Check sheet for the drawn part. Datum: minimum x, y, z corner. Units: mm. A direction names the side the tool comes from. Give positions to 0.01 mm unless a question says otherwise; leave off trailing zeros. Write each loop counter-clockwise with the first axis right and the second up, starting at its lowest first coordinate (ties: lowest second). Pieces come first, ordered by that corner, then holes.
(1) Cross-section at C-C (z = 51). Record the boundary of the cut face in (x, y).
(2) Cross-section at A-A (z = 5). Record the boundary of the cut face in (x, y), and give its area (3 significant figures).
(3) Thickness scan on line 1 along X through (y, z) = (1.55, 75); line 2 along Z through (x, y) = (5.25, 17.5); line 3 along Y through (x, z) = (6.25, 7.5). Record the ranges inside material, lowest first.
(4) Depth check by flat-ended pin: P1, Ø4.5, axis at y = 1, z = 13, coming from the -X side; P2, Ø1, axis at x = 8.5, y = 30, coming from the +Z side; P3, Ø8, axis at y = 33.5, z = 70, coming from the -X side. Enter the tip coordinate at first touch or a pass-through.
(5) Cross-section at D-D (y = 17). Record the boundary of the cut face in (x, z), and give its area (3 significant figures).
(6) Cross-section at B-B (x = 7.1). Record the boundary of the cut face in (y, z).
(7) Tool access check on the marked faces 1, 2 and 3. Record the directions out of +Z, -Z, +X, -X, +Y, -Y that give a thin tool (end or side, any length) a straight path to the whole face; none if there is none.
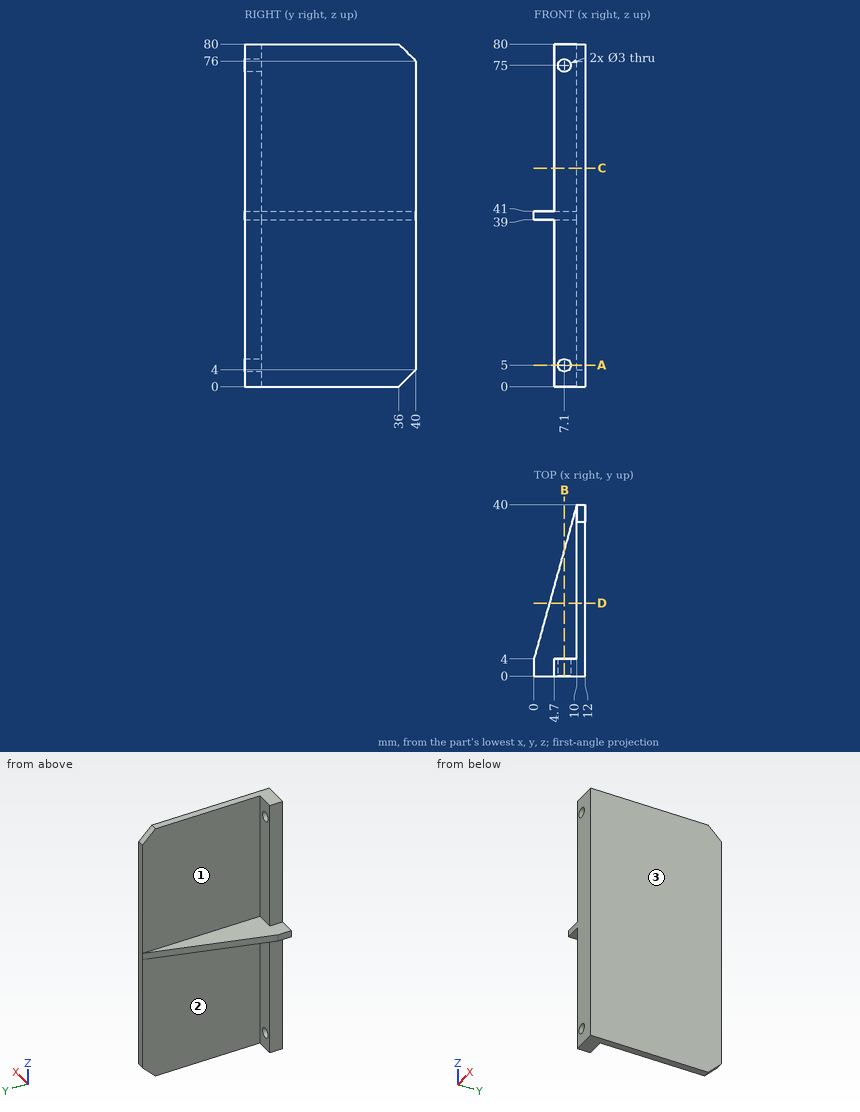
Reply:
1. outline: (4.7, 0) - (12, 0) - (12, 40) - (10, 40) - (10, 4) - (4.7, 4) - close
2. outline: (4.7, 0) - (5.6, 0) - (5.6, 4) - (4.7, 4) - close; (8.6, 0) - (12, 0) - (12, 40) - (10, 40) - (10, 4) - (8.6, 4) - close
2. area: 89.2 mm2
3. line 1: x = 4.7 to 5.6, 8.6 to 12
3. line 2: z = 39 to 41
3. line 3: y = 0 to 4
4. P1: stops at x = 4.7
4. P2: stops at z = 41
4. P3: stops at x = 10
5. outline: (3.61, 39) - (10, 39) - (10, 0) - (12, 0) - (12, 80) - (10, 80) - (10, 41) - (3.61, 41) - close
5. area: 173 mm2
6. outline: (0, 0) - (4, 0) - (4, 3.5) - (0, 3.5) - close; (0, 6.5) - (4, 6.5) - (4, 39) - (29.56, 39) - (29.56, 41) - (4, 41) - (4, 73.5) - (0, 73.5) - close; (0, 76.5) - (4, 76.5) - (4, 80) - (0, 80) - close
7. face 1: +Z, -X, +Y
7. face 2: -Z, -X, +Y
7. face 3: +Z, -Z, +X, +Y, -Y
